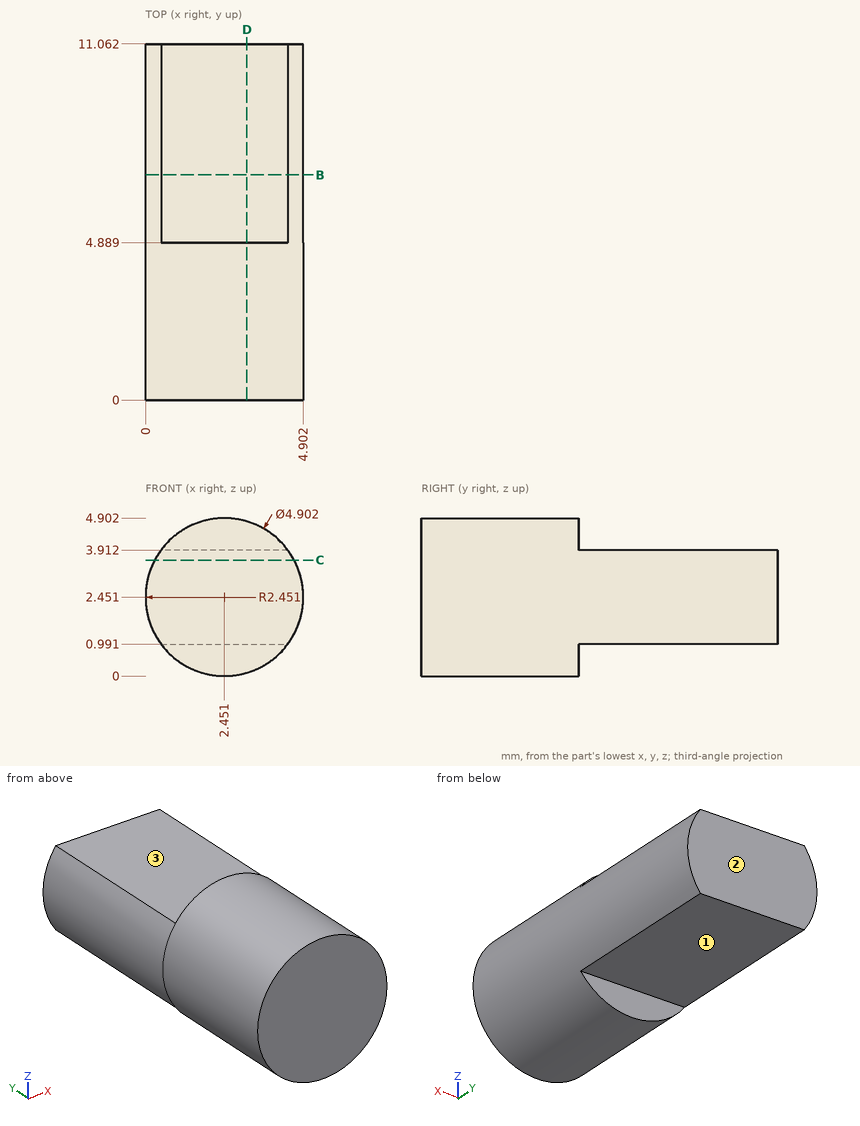
Input: dimensioned drawing with shaded views. Units: mm. Origin: part minimum x, y, z. A direction names the side the tool comes from. Round coordinates to 2 decimals unless told otherwise and drop trailing zeros. Order: outer loops, then holes, each group sorted by start corner. A loop starts at its lowest first (then second) coordinate and runs counter-clockwise, first axis right, second up. Notation, with made-up numbers: (51.25, 82) - (103.25, 82) arc R28 cw to (103.25, 119) - close; hole circle Ø8 at (3, 85). An arc over 180 degrees is marked (long way). Write item = value, one per line. Start each with the question number.
Q1. Cut plane D-D on x = 3.15. Return the cut outline in (y, z).
Q2. Cut plane B-B on y = 7. Return the cut outline in (x, z).
Q3. Cut plane C-C on z = 3.6. Return the cut outline in (x, y) (1 decimal).
Q4. Pin query (flat end, axial travel): pin 1 (0.8 mm diameter, centred on x = 3.5, z = 0.5, fed in from +Y); pin 2 (1.5 mm diameter, centred on x = 1.5, y = 4.5, fed in from +Z); pin 3 (2 mm diameter, centred on x = 1, y = 5, fed in from -Z). Return the tip coordinate at first contact, or that it passes through.
Q5. Access query for the marked faces 1, 2 and 3. Directions: +Z, -Z, +X, -X, +Y, -Y. A direction counts if a zero-diameter tool reaches every point of the face in a straight line with its end or side. Return the directions, or none.
Q6. Ray query, line 1 (Z direction, x = 3.6, y = 5); line 2 (Y direction, x = 2.2, z = 4.15); line 3 (Z direction, x = 4.6, y = 7.75) (1 decimal). Return the intervals inside material, ascending. Write a range as from..to.
Outcome:
q1.outline = (0, 0.1) - (4.89, 0.1) - (4.89, 0.99) - (11.06, 0.99) - (11.06, 3.91) - (4.89, 3.91) - (4.89, 4.8) - (0, 4.8) - close
q2.outline = (0.48, 0.99) - (4.42, 0.99) arc R2.45 ccw to (4.42, 3.91) - (0.48, 3.91) arc R2.45 ccw to start
q3.outline = (0.3, 0) - (4.6, 0) - (4.6, 11.1) - (0.3, 11.1) - close
q4.pin_1 = 4.89
q4.pin_2 = 4.89
q4.pin_3 = 0.04
q5.face_1 = -Z, +X, -X, +Y
q5.face_2 = +Z, -Z, +X, -X, +Y
q5.face_3 = +Z, +X, -X, +Y
q6.line_1 = 0.99..3.91
q6.line_2 = 0..4.89
q6.line_3 = 1.3..3.6
